Autodesk Inventor part; units mm, degrees
ref_plane "YZ Plane" through (0, 0, 0) normal (1, 0, 0) x (0, 1, 0)
ref_plane "XZ Plane" through (0, 0, 0) normal (0, 1, 0) x (-1, 0, 0)
ref_plane "XY Plane" through (0, 0, 0) normal (0, 0, 1) x (1, 0, 0)
sketch "Sketch1" plane through (0, 0, 0) normal (1, 0, 0) x (0, 1, 0)
  circle A0 centre (0, 0) radius 9.525
  circle A1 centre (0, 0) radius 8.7313
  line L0 (0, -9.525) -> (-12.7, -9.525)
  line L1 (-12.7, -9.525) -> (-12.7, -8.7313)
  line L2 (-12.7, -8.7313) -> (0, -8.7313)
  circle A2 centre (0, 0) radius 7.9375
  circle A3 centre (0, 0) radius 7.1438
  circle A4 centre (0, 0) radius 6.35
  point P0 (-3.8067, -8.7313)
  dimension "d13" = 19.05
  dimension "d0" = 0.7937
  dimension "d2" = 12.7
  dimension "d15" = 0.7937
  dimension "d16" = 0.7937
  dimension "d17" = 0.7937
extrude "Extrusion1" add sketch "Sketch1" along normal mid plane 12.7 contours A0 | L0 L1 L2 A0
chamfer "Chamfer2" distance 0.0254 angle 45 2 edges at (6.35, -8.7313, 0) (-6.35, -8.7313, 0)
extrude "Extrusion2" add sketch "Sketch1" along normal mid plane 12.7 contours A1
chamfer "Chamfer3" distance 0.0254 angle 45 4 edges at (-6.35, -8.7313, 0) (-6.35, -7.9375, 0) (6.35, -7.9375, 0) (6.35, -8.7313, 0)
extrude "Extrusion3" add sketch "Sketch1" along normal mid plane 12.7 contours A2
chamfer "Chamfer4" distance 0.0254 angle 45 4 edges at (-6.35, -7.9375, 0) (-6.35, -7.1438, 0) (6.35, -7.1438, 0) (6.35, -7.9375, 0)
extrude "Extrusion4" add sketch "Sketch1" along normal mid plane 12.7 contours A3
chamfer "Chamfer5" distance 0.0254 angle 45 1 edges at (-6.35, -7.1438, 0)
chamfer "Chamfer6" distance 0.127 angle 45 4 edges at (6.35, 1.9443, 9.3245) (6.35, -6.35, -9.525) (-6.35, 1.9443, 9.3245) (-6.35, -6.35, -9.525)
equation "\"d16\" = d15"
equation "\"d18\" = d3"
equation "\"d22\" = d8"
equation "\"d20\" = d3"
equation "\"d25\" = d8"
equation "\"d28\" = d3"
equation "\"d30\" = d8"
properties part number "GreyT Constant Force Spring" material "Steel"
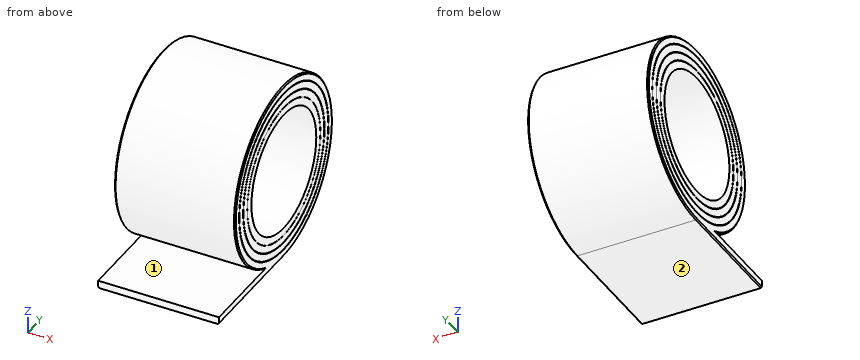
The model under review builds one solid part; all positions refer to its coordinate system, in mm. Face numbers are marked on the shaded views. Give positions to 0.01 mm unless a question says otherwise; leave off trailing zeros. Order: outer loops, then holes, each group sorted by start corner. A loop starts at its lowest first (then second) coordinate and runs counter-clockwise, first axis right, second up. Notation, with made-up numbers: M 32,68.5 L 56,68.5 A23 ccw 56,77.5 Z; hole C 7.25,-19 d8. An arc over 180 degrees is marked long. Use one line per item in the form item = value. Start each with the question number.
Item 1: We need section B-B on x = -2.25. Give the boundary of the cut face in (y, z) (3 decimals), plus the area to 3 significant figures.
Item 2: To check wall thickness, follow line 1 along Z through (x, y) = (2, 0) (3 decimals); line 2 along Z through (x, y) = (-4, -10.75) (3 decimals); line 3 along Z through (x, y) = (4.5, -3) (3 decimals). State the ranges of each line that lie inside material, in increasing order. Write a range as from..to.
Item 3: We need section A-A on y = -11. Give the boundary of the cut face in (x, z) (3 decimals).
Item 4: The part is to be moulded in two halves that separate along Z. For the marked faces 1 and 2, say which applies: pulls with the +Z half, pulls with the -Z half, needs draft (parallel to the pull), parting line crosses it, or undercut.
Item 5: Insertion check: pin 1 Ø4.5 at (x, y) = (-1.5, -9) entering from +Z; pin 2 Ø5 at (x, z) = (-3.5, 7.5) entering from +Y; pin 3 Ø1 at (x, y) = (4.5, 1) entering from +Z. Each pin has a flat end and moves straight along its axis. Give the tip position at first contact, or say it passes through.
Completed:
q1.outline = M -12.7,-9.525 L 0,-9.525 A9.525 ccw long -3.807,-8.731 L -12.7,-8.731 Z; hole C 0,0 d12.7
q1.area = 166 mm²
q2.line_1 = -9.525..-6.35, 6.35..9.525
q2.line_2 = -9.525..-8.731
q2.line_3 = -9.525..-5.597, 5.597..9.04
q3.outline = M -6.35,-9.398 L -6.223,-9.525 L 6.223,-9.525 L 6.35,-9.398 L 6.35,-8.731 L -6.35,-8.731 Z
q4.face_1 = undercut
q4.face_2 = pulls with the -Z half
q5.pin_1 = 6.72
q5.pin_2 = 8.11
q5.pin_3 = 9.51
